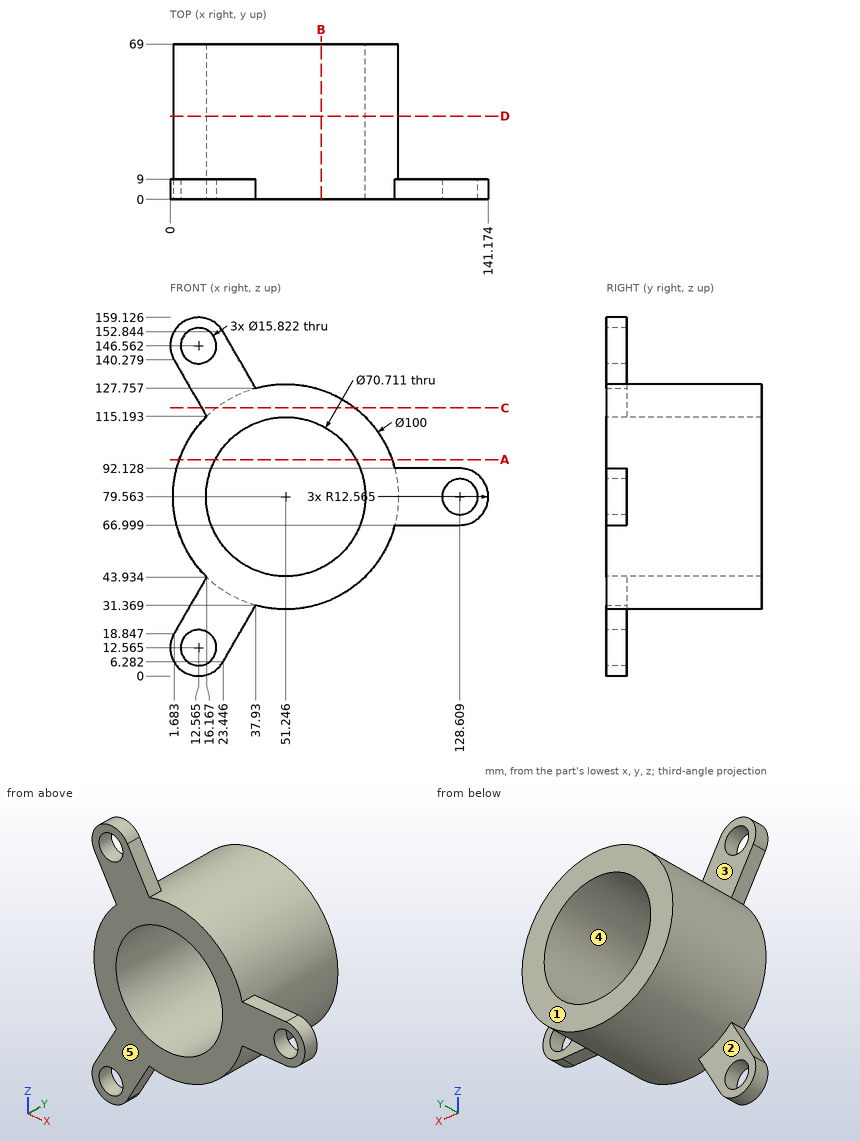
Study the drawing (mm; zero at the part's minimum x, y, z) and answer. A direction names the side the tool comes from. Give positions to 0.01 mm unless a question says otherwise; leave off trailing zeros. Write each loop counter-clockwise with the first axis right and the second up, starting at its lowest first coordinate (ties: lowest second). Pieces come first, ordered by that corner, then holes. Notation, with made-up numbers: (54, -19) -> (84, -19) arc R14 cw to (84, -14) -> close; hole circle Ø11 at (60, 80). An arc over 180 degrees is marked (long way). Answer in a Markdown table with one row per item.
1) Straight lines are drawn through the part: line 1 (Z direction, x = 50.5, y = 37) (1 decimal); line 2 (Z direction, x = 107, y = 5); line 3 (X direction, y = 13.5, z = 70) (1 decimal). For each, find the intervals that lie inside material, in ascending order. Write a range as [from, to].
Results list:
| item | result |
|---|---|
| line 1 | [29.6, 44.2], [114.9, 129.6] |
| line 2 | [67, 92.13] |
| line 3 | [2.2, 17.2], [85.3, 100.3] |
2) Section B-B on x = 67 is taken. Give the vertices of the cut face in (y, z) (1 decimal), plus the area to 3 significant figures.
Results list:
| item | result |
|---|---|
| outline | (0, 32.1) -> (69, 32.1) -> (69, 47.9) -> (0, 47.9) -> close; (0, 111.2) -> (69, 111.2) -> (69, 127) -> (0, 127) -> close |
| area | 2,180 mm^2 |
3) Each of these flat-tipped pins is pushed along its axis until it touches: pin 1 Ø4 at (x, y) = (57.5, 12.5) entering from -Z (1 decimal); pin 2 Ø4 at (y, z) = (54, 37.5) entering from -X; pin 3 Ø6 at (x, y) = (78, 56.5) entering from -Z (1 decimal). Where does it stop, or does it pass through?
Results list:
| item | result |
|---|---|
| pin 1 | z = 29.7 |
| pin 2 | x = 21.33 |
| pin 3 | z = 35.6 |
4) Section D-D on y = 37 is taken. Give the vertices of the cut face in (x, z) (1 decimal).
Results list:
| item | result |
|---|---|
| outline | circle Ø100 at (51.2, 79.6); hole circle Ø70.7 at (51.2, 79.6) |
5) Section A-A on z = 96 is taken. Give the vertices of the cut face in (x, y) (1 decimal).
Results list:
| item | result |
|---|---|
| outline | (4, 0) -> (19.9, 0) -> (19.9, 69) -> (4, 69) -> close; (82.5, 0) -> (98.5, 0) -> (98.5, 69) -> (82.5, 69) -> close |
6) Section C-C on z = 119 is taken. Give the vertices of the cut face in (x, y).
Results list:
| item | result |
|---|---|
| outline | (13.97, 0) -> (81.98, 0) -> (81.98, 69) -> (20.51, 69) -> (20.51, 9) -> (13.97, 9) -> close |
7) A tool of negligible diameter and unlimited length cuts with its end or side. For the marked faces 1, 2 and 3, from which of +Z, -Z, +X, -X, +Y, -Y can it reach the whole face along a straight path? Write none if from no direction.
Results list:
| item | result |
|---|---|
| face 1 | +Z, -Z, +X, -X, +Y |
| face 2 | -Z, -X, +Y |
| face 3 | +Z, -X, +Y |
8) Determine the mould class of the marked faces 4 and 5 for opening direction X: released by +X, released by -X, zero draft, split by the parting line, or undercut.
Results list:
| item | result |
|---|---|
| face 4 | undercut |
| face 5 | zero draft |
